```python
from build123d import *

# Parameters (mm, degrees)
SKETCH1_W               = 175
SKETCH1_H               = 175
BOSS_EXTRUDE1_DEPTH     = 5
SKETCH3_W               = 145
SKETCH3_H               = 6
BOSS_EXTRUDE3_DEPTH     = 18
SKETCH4_R               = 2
CUT_EXTRUDE2_DEPTH      = 1
CUT_EXTRUDE2_DEPTH_BACK = 176
SKETCH5_W               = 10
SKETCH5_H               = 115
CUT_EXTRUDE3_DEPTH      = 10


with BuildPart() as part:
    # Sketch1 → Boss-Extrude1 (new body)
    with BuildSketch(Plane(origin=(0, 0, 0), x_dir=(1, 0, 0), z_dir=(0, 1, 0))):
        with Locations((-24.045801527, -27.385496183)):
            Rectangle(SKETCH1_W, SKETCH1_H)
    extrude(amount=BOSS_EXTRUDE1_DEPTH)

    # Sketch3 → Boss-Extrude3 (add)
    with BuildSketch(Plane.XZ):
        with Locations((-24.045801527, 111.885496183)):
            Rectangle(SKETCH3_W, SKETCH3_H)
        with Locations((-24.045801527, -57.114503817)):
            Rectangle(SKETCH3_W, SKETCH3_H)
    extrude(amount=BOSS_EXTRUDE3_DEPTH)

    # Sketch4 → Cut-Extrude2 (cut, two sides)
    with BuildSketch(Plane(origin=(0, 0, -60.114503817), x_dir=(-1, 0, 0), z_dir=(0, 0, -1))) as cut_extrude2_sk:
        with Locations((-28.454198473, -8.900832872)):
            Circle(SKETCH4_R)
        with Locations((24.045801527, -8.900832872)):
            Circle(SKETCH4_R)
        with Locations((76.545801527, -8.900832872)):
            Circle(SKETCH4_R)
    extrude(amount=CUT_EXTRUDE2_DEPTH, mode=Mode.SUBTRACT)
    extrude(cut_extrude2_sk.sketch, amount=-CUT_EXTRUDE2_DEPTH_BACK, mode=Mode.SUBTRACT)

    # Sketch5 → Cut-Extrude3 (cut)
    with BuildSketch(Plane(origin=(0, 5, 0), x_dir=(1, 0, 0), z_dir=(0, 1, 0))):
        with Locations((-106.545801527, -27.385496183)):
            Rectangle(SKETCH5_W, SKETCH5_H)
        with Locations((58.454198473, -27.385496183)):
            Rectangle(SKETCH5_W, SKETCH5_H)
    extrude(amount=-CUT_EXTRUDE3_DEPTH, mode=Mode.SUBTRACT)


solid = part.part
```
Here's how the part is built. I have some questions about the finished solid (model axes, mm). A direction names the side the tool comes from. Round coordinates to 2 decimals unless told otherwise and drop trailing zeros. Write each loop counter-clockwise with the first axis right and the second up, starting at its lowest first coordinate (ties: lowest second). Pieces come first, ordered by that corner, then holes. Notation, with made-up numbers: M 29,21 L 35,21 A11 ccw 35,25 Z; hole C 68.5,-8 d5. An arc over 180 degrees is marked long. Answer as CSV lines item,"result". Start each with the question number.
1. I'm going to push flat-ended pins straight in: pin 1 Ø2 at (x, z) = (-73, 50.5) entering from -Y; pin 2 Ø5 at (x, y) = (-24.05, -8.9) entering from -Z; pin 3 Ø5 at (y, z) = (-12, -56) entering from -X; pin 4 Ø6.5 at (y, z) = (-11, 112.5) entering from +X. Where does each tip first touch, or does it pass through?
2. On a 3-axis mill with a long thin cutter (end or side, diameter ignored), from which of +Z, -Z, +X, -X, +Y, -Y can I reach the whole of each face in a straight line? I mean faces 1 (the flat face through (-25, -18, -57)), 2 (the cylindrical face through (-74.548, -8.813, 111.843)), 3 (the flat face through (-96.546, -9, 112)), 4 (the flat face through (48.454, -9, 112)), 5 (the flat face through (-101.546, 3, 28)). Say none if no direction works.
3. Suppose I cut it at D-D on z = -38. Write out the boundary of the cut face in (x, y), then the cut area to 3 significant figures.
4. Suppose I cut it at C-C on z = -4. Write out the boundary of the cut face in (x, y).
5. Suppose I cut it at A-A on y = -2.5. Write out the boundary of the cut face in (x, z), then the cut area to 3 significant figures.
6. Thinking about a two-plate mould opening in Z: for faces 6 (the flat face through (-25, -11, 108.885)), 7 (the flat face through (-96.546, -9, -57)), 8 (the flat face through (53.454, 3, 28)), which applies, released by +Z, released by -Z, zero draft, split by the parting line, or undercut?
7. I need wall thicknesses on probe 1 along Z at (x, y) = (7, -4.5); probe 2 along X at (y, z) = (2.5, 73.5); probe 3 along Y at (x, z) = (11, -15.5). Which ranges of each line are inside material? Lowest first, please.
8. Suppose I cut it at B-B on x = 22.5. Write out the boundary of the cut face in (y, z).
Check result:
1,pin 1,"stops at y = 0"
1,pin 2,"stops at z = -60.11"
1,pin 3,"stops at x = -96.55"
1,pin 4,"stops at x = 48.45"
2,face 1,"+Z, -Z, +X, -X, -Y"
2,face 2,"+Z, -Z"
2,face 3,"+Z, -Z, -X, -Y"
2,face 4,"+Z, -Z, +X, -Y"
2,face 5,"-X, +Y, -Y"
3,outline,"M -111.55,0 L 63.45,0 L 63.45,5 L -111.55,5 Z"
3,area,"875 mm2"
4,outline,"M -101.55,0 L 53.45,0 L 53.45,5 L -101.55,5 Z"
5,outline,"M -96.55,-60.11 L 48.45,-60.11 L 48.45,-54.11 L -96.55,-54.11 Z; M -96.55,108.89 L 48.45,108.89 L 48.45,114.89 L -96.55,114.89 Z"
5,area,"1,740 mm2"
6,face 6,"undercut"
6,face 7,"zero draft"
6,face 8,"undercut"
7,probe 1,"z = -60.11 to -54.11, 108.89 to 114.89"
7,probe 2,"x = -101.55 to 53.45"
7,probe 3,"y = 0 to 5"
8,outline,"M -18,-60.11 L 5,-60.11 L 5,114.89 L -18,114.89 L -18,108.89 L 0,108.89 L 0,-54.11 L -18,-54.11 Z"
